from build123d import *
from build123d import SkipClean  # not in build123d's __all__

# Parameters (mm, degrees)
F0_R            = 12.7
F1_DEPTH        = 35.56
F2_R            = 8.255
F3_DEPTH        = 9.525
F4_R            = 2.667
F5_DEPTH        = 254
F9_DEPTH        = 25.4
F9_COPIES_COUNT = 3
F10_R           = 1.27
F6_R            = 8.255
F6_R_2          = 2.667
F11_DEPTH       = 15.748


# Not quite as in the source:
# - a pattern or mirror of a feature is missing from the dataset's text; its kind, count and spacing are read off the source's solid
# - a feature names something its author has since deleted; it is built from what else it names


with BuildPart() as f1:
    # F0 (on Top) → F1 (new body)
    with BuildSketch(Plane.XY):
        Circle(F0_R)
    extrude(amount=F1_DEPTH)

    # F2 (on face) → F3 (cut)
    with BuildSketch(Plane.XY.offset(35.56)):
        Circle(F2_R)
    extrude(amount=-F3_DEPTH, mode=Mode.SUBTRACT)

    # F4 (on face) → F5 (cut)
    with BuildSketch(Plane.XY.offset(26.035)):
        Circle(F4_R)
    extrude(amount=-F5_DEPTH, mode=Mode.SUBTRACT)

    # F8 (on offset) → F9 (join)
    with BuildSketch(Plane.YZ.offset(7.62)):
        with BuildLine():
            Line((-7.096601933, 1.1829776548), (-6.096, 0))
            add(Edge.make_bspline(
                [(-6.096, 0), (-5.8943346547, 1.9452293607), (-5.4834307395, 5.9087381092), (0.5997187932, 8.6736721856), (1.7285446911, 11.9368345808), (2.2646340076, 13.4865390137)],
                knots=[0, 0, 0, 0, 0.3360272787, 0.6846735329, 1, 1, 1, 1], degree=3))
            Line((2.2646340076, 13.4865390137), (1.47131423, 14.712578617))
            add(Edge.make_bspline(
                [(-7.096601933, 1.1829776548), (-6.9020267489, 2.8395199903), (-6.4802421103, 6.4304409685), (-0.1009646663, 10.0195226908), (0.978146166, 13.2405336059), (1.47131423, 14.712578617)],
                knots=[0, 0, 0, 0, 0.3174047687, 0.6880448619, 1, 1, 1, 1], degree=3))
        make_face()
    with SkipClean():  # cleaning this boolean's faces spoils the solid; the shape is the same uncleaned
        f9 = extrude(amount=F9_DEPTH)

    # F9_copies: F9 ×3 about axis
    f9_copies_axis = Axis((0, 0, 0), (0, 0, 1))
    for i in range(1, F9_COPIES_COUNT):
        add(f9.rotate(f9_copies_axis, i * 360 / F9_COPIES_COUNT), clean=False)

    # F10
    f10_edges = [f1.edges().sort_by_distance(p)[0] for p in [
        (33.02, -6.596301, 0.591489),
    ]]
    fillet(f10_edges, radius=F10_R)

    # F6 (on face) → F11 (cut)
    with BuildSketch(Plane(origin=(0, 0, 0), x_dir=(1, 0, 0), z_dir=(0, 0, -1))):
        Circle(F6_R)
        Circle(F6_R_2, mode=Mode.SUBTRACT)
    extrude(amount=-F11_DEPTH, mode=Mode.SUBTRACT)


solid = f1.part
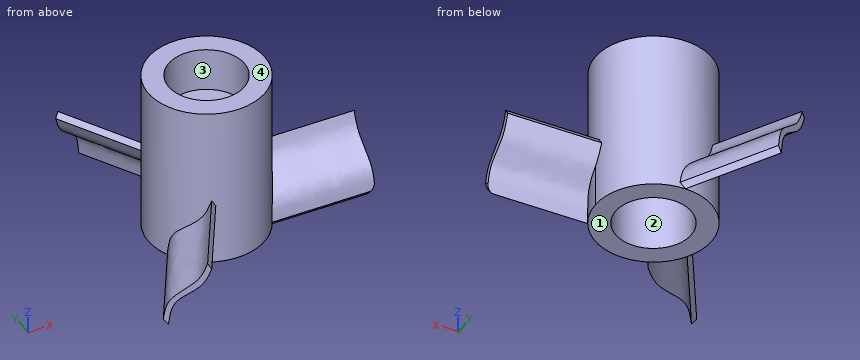
Could you check a few things on this model? Use its own coordinates, in mm. Face numbers are marked on the shaded views. A direction names the side the tool comes from. Round coordinates to 2 decimals unless told otherwise and drop trailing zeros. Write each loop counter-clockwise with the first axis right and the second up, starting at its lowest first coordinate (ties: lowest second). Pieces come first, ordered by that corner, then holes. Notation, with made-up numbers: (23, 30) - (82, 30) arc R20 ccw to (82, 46) - close; hole circle Ø4 at (45.5, -3). An arc over 180 degrees is marked (long way). Use a Markdown table: item, result.
Q1. For the marked faces 1 and 2, which set-ups out of +Z, -Z, +X, -X, +Y, -Y let a thin tool reach every point of the face, with its end or its side?
Output values:
| item | result |
|---|---|
| face 1 | -Z, +X, -X, +Y, -Y |
| face 2 | -Z |
Q2. For pin 1 (5 mm diameter, centred on x = -0.5, y = 1, fed in from -Z); pin 2 (1.5 mm diameter, centred on y = -6, z = 25, fed in from +X); pin 3 (8.5 mm diameter, centred on x = -3, y = 2.5, fed in from +Z) (3 decimals), each with a flat end and sliding along its axis, tell me the tip position at first contact or that it passes through.
Output values:
| item | result |
|---|---|
| pin 1 | z = 15.75 |
| pin 2 | x = 11.56 |
| pin 3 | z = 26.035 |
Q3. Please list where these lines run through material, in increasing order: L1, parallel to X at y = 0, z = 19; L2, parallel to Y at x = 0, z = 32 (3 decimals).
Output values:
| item | result |
|---|---|
| L1 | -12.7 to -2.67, 2.67 to 12.7 |
| L2 | -12.7 to -8.255, 8.255 to 12.7 |
Q4. Thinking about a two-plate mould opening in Y: for the marked faces 3 and 4, which applies, released by +Y, released by -Y, zero draft, split by the parting line, or undercut?
Output values:
| item | result |
|---|---|
| face 3 | undercut |
| face 4 | zero draft |
Q5. I want a section at B-B (x = 3.5). List the corners of the cut face in (y, z) for me (3 decimals), plus the area to 3 significant figures.
Output values:
| item | result |
|---|---|
| outline | (-12.208, 0) - (-7.476, 0) - (-7.476, 15.748) - (7.476, 15.748) - (7.476, 0) - (12.208, 0) - (12.208, 35.56) - (7.476, 35.56) - (7.476, 26.035) - (-7.476, 26.035) - (-7.476, 35.56) - (-12.208, 35.56) - close |
| area | 490 mm2 |
Q6. I want a section at C-C (z = 21.5). List the corners of the cut face in (x, y) for me.
Output values:
| item | result |
|---|---|
| outline | circle Ø25.4 at (0, 0); hole circle Ø5.33 at (0, 0) |
Q7. I want a section at A-A (z = 33). List the corners of the cut face in (x, y) for me (3 decimals), plus the area to 3 significant figures.
Output values:
| item | result |
|---|---|
| outline | circle Ø25.4 at (0, 0); hole circle Ø16.51 at (0, 0) |
| area | 293 mm2 |
